Read the model definition and answer for the solid it produces. Units are mm, in the model's axes. Face numbers are marked on the shaded views. Round coordinates to 2 decimals unless told otherwise and drop trailing zeros. Write each loop counter-clockwise with the first axis right and the second up, starting at its lowest first coordinate (ties: lowest second). Pieces come first, ordered by that corner, then holes. Notation, with made-up numbers: (73, 88) -> (91, 88) arc R31 cw to (91, 116) -> close; hole circle Ø7 at (69, 21.5). An arc over 180 degrees is marked (long way). Return JSON: item names as keys, results as strings.
from build123d import *

# Parameters (mm, degrees)
SKETCH1_W           = 7
SKETCH1_H           = 7
SKETCH1_R           = 2
SKETCH1_R_2         = 2.5
SKETCH1_H_2         = 7.25
SKETCH1_R_3         = 2.502389359
BOSS_EXTRUDE1_DEPTH = 2.5


with BuildPart() as part:
    # Sketch1 → Boss-Extrude1 (new body)
    with BuildSketch(Plane(origin=(0, 0, 0), x_dir=(1, 0, 0), z_dir=(0, 1, 0))):
        Polygon((-45.382608696, 29.153623188), (-80.382608696, 29.153623188), (-80.382608696, 25.653623188), (-80.382608696, 16.653623188), (-80.382608696, 4.153623188), (-80.382608696, -15.846376812), (-80.382608696, -28.346376812), (-80.382608696, -37.346376812), (-80.382608696, -40.846376812), (33.417391304, -40.846376812), (33.417391304, -5.846376812), (33.417391304, 29.153623188), (15.417391304, 29.153623188), (-37.582608696, 29.153623188), align=None)
        with Locations((-66.92185538, -33.846376812)):
            Rectangle(SKETCH1_W, SKETCH1_H, mode=Mode.SUBTRACT)
        with Locations(Location((-76.382608696, -28.346376812, 0), (0, 0, 270))):
            Circle(SKETCH1_R, mode=Mode.SUBTRACT)
        with Locations(Location((-49.382608696, -28.346376812, 0), (0, 0, 270))):
            Circle(SKETCH1_R, mode=Mode.SUBTRACT)
        with Locations(Location((-37.582608696, -14.846376812, 0), (0, 0, 270))):
            Circle(SKETCH1_R_2, mode=Mode.SUBTRACT)
        with Locations((-10.97764978, -33.721376812)):
            Rectangle(SKETCH1_W, SKETCH1_H_2, mode=Mode.SUBTRACT)
        with Locations(Location((15.417391304, -30.096376812, 0), (0, 0, 270))):
            Circle(SKETCH1_R_2, mode=Mode.SUBTRACT)
        with Locations(Location((-0.082608696, -5.846376812, 0), (0, 0, 270))):
            Circle(SKETCH1_R, mode=Mode.SUBTRACT)
        with Locations(Location((-76.382608696, 16.653623188, 0), (0, 0, 270))):
            Circle(SKETCH1_R, mode=Mode.SUBTRACT)
        Polygon((-70.47764978, 18.653623188), (-70.47764978, 25.653623188), (-70.42185538, 25.653623188), (-63.47764978, 25.653623188), (-63.47764978, 18.653623188), (-70.42185538, 18.653623188), align=None, mode=Mode.SUBTRACT)
        with Locations(Location((-49.382608696, 16.653623188, 0), (0, 0, 270))):
            Circle(SKETCH1_R, mode=Mode.SUBTRACT)
        with Locations(Location((-37.582608696, 13.153623188, 0), (0, 0, 270))):
            Circle(SKETCH1_R_2, mode=Mode.SUBTRACT)
        with Locations(Location((27.917391304, -5.846376812, 0), (0, 0, 270))):
            Circle(SKETCH1_R_3, mode=Mode.SUBTRACT)
        with Locations((-10.97764978, 22.153623188)):
            Rectangle(SKETCH1_W, SKETCH1_H, mode=Mode.SUBTRACT)
        with Locations(Location((15.417391304, 18.403623188, 0), (0, 0, 270))):
            Circle(SKETCH1_R_2, mode=Mode.SUBTRACT)
    extrude(amount=BOSS_EXTRUDE1_DEPTH)


solid = part.part
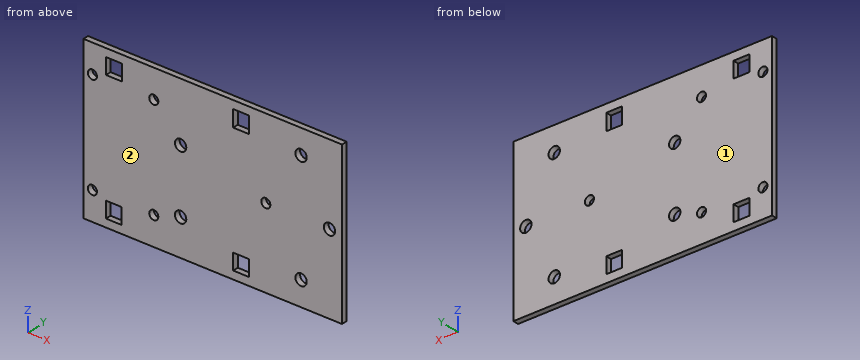
Item 1: Section C-C (y = 1.8) is taken. State how many separate pieces and enclosed holes the cut face has, then the cut area to 3 significant figures.
Worked answers:
{"separate pieces": "1", "enclosed holes": "14", "area": "7,610 mm2"}
Item 2: Straight lines are drawn through the part: L1, parallel to X at y = 2.3, z = -23; L2, parallel to Z at x = -68, y = 1.3; L3, parallel to Z at x = -14, y = 2.15. For each, find the intervals that lie inside material, in ascending order. Write a range as [from, to].
Worked answers:
{"L1": "x = [-80.38, -70.48], [-63.48, -14.48], [-7.48, 33.42]", "L2": "z = [-29.15, -25.65], [-18.65, 30.35], [37.35, 40.85]", "L3": "z = [-29.15, -25.65], [-18.65, 30.1], [37.35, 40.85]"}
Item 3: Section B-B (z = -23) is taken. Give the vertices of the cut face in (x, y), then the cut area to 4 significant figures.
Worked answers:
{"outline": "(-80.38, 0) -> (-70.48, 0) -> (-70.48, 2.5) -> (-80.38, 2.5) -> close; (-63.48, 0) -> (-14.48, 0) -> (-14.48, 2.5) -> (-63.48, 2.5) -> close; (-7.48, 0) -> (33.42, 0) -> (33.42, 2.5) -> (-7.48, 2.5) -> close", "area": "249.5 mm2"}
Item 4: For a pull along Y with two mould halves and no side action, classify the marked faces 1 and 2 as released by +Y, released by -Y, zero draft, split by the parting line, or undercut.
Worked answers:
{"face 1": "released by +Y", "face 2": "released by -Y"}
Item 5: Section A-A (x = -65) is taken. Give the vertices of the cut face in (y, z).
Worked answers:
{"outline": "(0, -29.15) -> (2.5, -29.15) -> (2.5, -25.65) -> (0, -25.65) -> close; (0, -18.65) -> (2.5, -18.65) -> (2.5, 30.35) -> (0, 30.35) -> close; (0, 37.35) -> (2.5, 37.35) -> (2.5, 40.85) -> (0, 40.85) -> close"}
